```python
from build123d import *

# Parameters (mm, degrees)
SKETCH_1_W           = 206.744673609
SKETCH_1_H           = 106.97480061
EXTRUDE_1_DEPTH      = 3
SKETCH_3_W           = 200.744673609
SKETCH_3_H           = 100.97480061
EXTRUDE_2_DEPTH      = 22.6000508
SKETCH_4_W           = 18
SKETCH_4_H           = 10
CUT_EXTRUDE_1_DEPTH  = 5
SKETCH_6_W           = 16
SKETCH_6_H           = 16
CUT_EXTRUDE_2_DEPTH  = 5
SKETCH_7_W           = 16
SKETCH_7_H           = 16
CUT_EXTRUDE_3_DEPTH  = 5
SKETCH_8_W           = 18
SKETCH_8_H           = 10
CUT_EXTRUDE_4_DEPTH  = 5
SKETCH_9_W           = 35.828584262
SKETCH_9_H           = 13.394073463
CUT_EXTRUDE_5_DEPTH  = 5
SKETCH_10_R          = 3.719289999
CUT_EXTRUDE_6_DEPTH  = 5
SKETCH_11_W          = 9.469470229
SKETCH_11_H          = 12.194282659
CUT_EXTRUDE_7_DEPTH  = 5
SKETCH_12_R          = 3.134321658
CUT_EXTRUDE_8_DEPTH  = 5
SKETCH_13_R          = 1.6
CUT_EXTRUDE_9_DEPTH  = 5
SKETCH_15_W          = 25
SKETCH_15_H          = 20
CUT_EXTRUDE_11_DEPTH = 1.5
SKETCH_16_W          = 20
SKETCH_16_H          = 70
CUT_EXTRUDE_12_DEPTH = 1.5
FILLET_1_R           = 1.5
SKETCH_17_W          = 18.030255685
SKETCH_17_H          = 1.793339536
SKETCH_17_W_2        = 18.10659189
SKETCH_17_W_3        = 18.089855477
SKETCH_17_W_4        = 17.999756417
SKETCH_17_W_5        = 18.030454167
CUT_EXTRUDE_13_DEPTH = 6.89172601
SKETCH_18_W          = 18.338169952
SKETCH_18_H          = 1.939199609
CUT_EXTRUDE_14_DEPTH = 7.158781029
SKETCH_21_W          = 7.461807672
SKETCH_21_H          = 3.5
SKETCH_21_W_2        = 3.5
SKETCH_21_H_2        = 6.158755504
SKETCH_21_H_3        = 6.106655877
SKETCH_21_H_4        = 6.247919092
CUT_EXTRUDE_16_DEPTH = 13


with BuildPart() as part:
    # 草图1 → 凸台-拉伸1 (new body)
    with BuildSketch(Plane(origin=(0, 0, -6), x_dir=(-1, 0, 0), z_dir=(0, 0, -1))):
        with Locations((-142.557122174, -194.856389383)):
            Rectangle(SKETCH_1_W, SKETCH_1_H)
    extrude(amount=EXTRUDE_1_DEPTH)

    # 草图3 → 凸台-拉伸2 (add)
    with BuildSketch(Plane.XY.offset(-6)):
        Polygon((39.18478537, -141.368989078), (245.929458979, -141.368989078), (245.929458979, -248.343789688), (39.18478537, -248.343789688), (39.18478537, -243.18233024), (39.18478537, -146.483402372), align=None)
        with Locations((142.557122174, -194.856389383)):
            Rectangle(SKETCH_3_W, SKETCH_3_H, mode=Mode.SUBTRACT)
    extrude(amount=EXTRUDE_2_DEPTH)

    # 草图4 → 切除-拉伸1 (cut)
    with BuildSketch(Plane.XZ.offset(248.343789688)):
        with Locations((105.2106038, 4.708324791)):
            Rectangle(SKETCH_4_W, SKETCH_4_H)
        with Locations((63.5106038, 4.708324791)):
            Rectangle(SKETCH_4_W, SKETCH_4_H)
        with Locations((147.8106038, 4.708324791)):
            Rectangle(SKETCH_4_W, SKETCH_4_H)
        with Locations((190.5106038, 4.708324791)):
            Rectangle(SKETCH_4_W, SKETCH_4_H)
        with Locations((233.2106038, 4.708324791)):
            Rectangle(SKETCH_4_W, SKETCH_4_H)
    extrude(amount=-CUT_EXTRUDE_1_DEPTH, mode=Mode.SUBTRACT)

    # 草图6 → 切除-拉伸2 (cut)
    with BuildSketch(Plane(origin=(245.929458979, 0, 0), x_dir=(0, 0, -1), z_dir=(1, 0, 0))):
        with Locations((-6.6000508, -220.799301723)):
            Rectangle(SKETCH_6_W, SKETCH_6_H)
        with Locations((-6.6000508, -197.299301723)):
            Rectangle(SKETCH_6_W, SKETCH_6_H)
        with Locations((-6.6000508, -173.799301723)):
            Rectangle(SKETCH_6_W, SKETCH_6_H)
    extrude(amount=-CUT_EXTRUDE_2_DEPTH, mode=Mode.SUBTRACT)

    # 草图7 → 切除-拉伸3 (cut)
    with BuildSketch(Plane(origin=(0, -141.368989078, 0), x_dir=(1, 0, 0), z_dir=(0, 1, 0))):
        with Locations((226.905896319, -6.6000508)):
            Rectangle(SKETCH_7_W, SKETCH_7_H)
    extrude(amount=-CUT_EXTRUDE_3_DEPTH, mode=Mode.SUBTRACT)

    # 草图8 → 切除-拉伸4 (cut)
    with BuildSketch(Plane(origin=(0, -141.368989078, 0), x_dir=(1, 0, 0), z_dir=(0, 1, 0))):
        with Locations((143.087906607, -4.441269771)):
            Rectangle(SKETCH_8_W, SKETCH_8_H)
    extrude(amount=-CUT_EXTRUDE_4_DEPTH, mode=Mode.SUBTRACT)

    # 草图9 → 切除-拉伸5 (cut)
    with BuildSketch(Plane(origin=(0, -141.368989078, 0), x_dir=(1, 0, 0), z_dir=(0, 1, 0))):
        with Locations((193.834394064, -4.192873823)):
            Rectangle(SKETCH_9_W, SKETCH_9_H)
    extrude(amount=-CUT_EXTRUDE_5_DEPTH, mode=Mode.SUBTRACT)

    # 草图10 → 切除-拉伸6 (cut)
    with BuildSketch(Plane(origin=(0, -141.368989078, 0), x_dir=(1, 0, 0), z_dir=(0, 1, 0))):
        with Locations(Location((101.045841124, -4.188653157, 0), (0, 0, 270))):
            Circle(SKETCH_10_R)
    extrude(amount=-CUT_EXTRUDE_6_DEPTH, mode=Mode.SUBTRACT)

    # 草图11 → 切除-拉伸7 (cut)
    with BuildSketch(Plane(origin=(0, -141.368989078, 0), x_dir=(1, 0, 0), z_dir=(0, 1, 0))):
        with Locations((57.128440025, -10.502909471)):
            Rectangle(SKETCH_11_W, SKETCH_11_H)
    extrude(amount=-CUT_EXTRUDE_7_DEPTH, mode=Mode.SUBTRACT)

    # 草图12 → 切除-拉伸8 (cut)
    with BuildSketch(Plane.ZY.offset(-39.18478537)):
        with Locations((4.250612207, -173.693029578)):
            Circle(SKETCH_12_R)
        with Locations((4.250612207, -197.243029578)):
            Circle(SKETCH_12_R)
        with Locations((4.250612207, -220.793029578)):
            Circle(SKETCH_12_R)
    extrude(amount=-CUT_EXTRUDE_8_DEPTH, mode=Mode.SUBTRACT)

    # 草图13 → 切除-拉伸9 (cut)
    with BuildSketch(Plane(origin=(0, 0, -9), x_dir=(-1, 0, 0), z_dir=(0, 0, -1))):
        with Locations((-238.585543847, -149.289415757)):
            Circle(SKETCH_13_R)
        with Locations((-46.99814318, -148.85706783)):
            Circle(SKETCH_13_R)
        with Locations((-46.669564212, -229.041899724)):
            Circle(SKETCH_13_R)
        with Locations((-239.137231318, -229.121228359)):
            Circle(SKETCH_13_R)
    extrude(amount=-CUT_EXTRUDE_9_DEPTH, mode=Mode.SUBTRACT)

    # 草图15 → 切除-拉伸11 (cut)
    with BuildSketch(Plane(origin=(0, -141.368989078, 0), x_dir=(1, 0, 0), z_dir=(0, 1, 0))):
        with Locations((101.081540793, -4.6000508)):
            Rectangle(SKETCH_15_W, SKETCH_15_H)
    extrude(amount=-CUT_EXTRUDE_11_DEPTH, mode=Mode.SUBTRACT)

    # 草图16 → 切除-拉伸12 (cut)
    with BuildSketch(Plane.ZY.offset(-39.18478537)):
        with Locations((4.6000508, -197.704987162)):
            Rectangle(SKETCH_16_W, SKETCH_16_H)
    extrude(amount=-CUT_EXTRUDE_12_DEPTH, mode=Mode.SUBTRACT)

    # 圆角1
    fillet_1_edges = [part.edges().sort_by_distance(p)[0] for p in [
        (245.929458979, -141.368989078, 3.8000254),
        (39.18478537, -141.368989078, 3.8000254),
        (39.18478537, -248.343789688, 3.8000254),
        (245.929458979, -248.343789688, 3.8000254),
    ]]
    fillet(fillet_1_edges, radius=FILLET_1_R)

    # 草图17 → 切除-拉伸13 (cut)
    with BuildSketch(Plane.XY.offset(16.6000508)):
        with Locations((63.500922097, -246.240459456)):
            Rectangle(SKETCH_17_W, SKETCH_17_H)
        with Locations((105.179998956, -246.240459456)):
            Rectangle(SKETCH_17_W_2, SKETCH_17_H)
        with Locations((147.809231135, -246.240459456)):
            Rectangle(SKETCH_17_W_3, SKETCH_17_H)
        with Locations((190.556004567, -246.240459456)):
            Rectangle(SKETCH_17_W_4, SKETCH_17_H)
        with Locations((233.233676321, -246.240459456)):
            Rectangle(SKETCH_17_W_5, SKETCH_17_H)
    extrude(amount=-CUT_EXTRUDE_13_DEPTH, mode=Mode.SUBTRACT)

    # 草图18 → 切除-拉伸14 (cut)
    with BuildSketch(Plane.XY.offset(16.6000508)):
        with Locations((143.227232083, -143.399389273)):
            Rectangle(SKETCH_18_W, SKETCH_18_H)
    extrude(amount=-CUT_EXTRUDE_14_DEPTH, mode=Mode.SUBTRACT)

    # 草图21 → 切除-拉伸16 (cut)
    with BuildSketch(Plane.XY.offset(16.6000508)):
        with Locations((101.01663333, -143.118989078)):
            Rectangle(SKETCH_21_W, SKETCH_21_H)
        with Locations((40.93478537, -173.649755278)):
            Rectangle(SKETCH_21_W_2, SKETCH_21_H_2)
        with Locations((40.93478537, -197.254331907)):
            Rectangle(SKETCH_21_W_2, SKETCH_21_H_3)
        with Locations((40.93478537, -220.776300492)):
            Rectangle(SKETCH_21_W_2, SKETCH_21_H_4)
    extrude(amount=-CUT_EXTRUDE_16_DEPTH, mode=Mode.SUBTRACT)


solid = part.part
```
The model under review builds one solid part; all positions refer to its coordinate system, in mm. A direction names the side the tool comes from. Round coordinates to 2 decimals unless told otherwise and drop trailing zeros. Loops run counter-clockwise (first coordinate to the right, second up) from the corner with the lowest first, then second, coordinate; pieces in that order, holes last. Notation, with made-up numbers: M -36.75,38.25 L 5.25,38.25 A22 ccw 5.25,50.25 Z; hole C 14.5,-27.75 d6. An arc over 180 degrees is marked long. Write item = value, one per line.
Item 1: Take a section at D-D on y = -220. Write out the cut boundary in (x, z).
Return value:
outline = M 39.18,-9 L 245.93,-9 L 245.93,-1.4 L 242.93,-1.4 L 242.93,-6 L 42.18,-6 L 42.18,1.22 L 40.68,1.22 L 40.68,-5.4 L 39.18,-5.4 Z; M 242.93,14.6 L 245.93,14.6 L 245.93,16.6 L 242.93,16.6 Z
Item 2: For line 1 (X direction, y = -243, z = 13.25); line 2 (Y direction, x = 156, z = -3.75); line 3 (Y direction, x = 91.5, z = -2.25), list the stretches that pass through material, from the lowest coordinate up. Write a range as [from, to].
Return value:
line_1 = [39.18, 42.18], [242.93, 245.93]
line_2 = [-248.34, -245.34], [-144.37, -141.37]
line_3 = [-248.34, -245.34], [-144.37, -142.87]
Item 3: Insertion check: P1, Ø0.9, axis at x = 40.5, z = 11.5, coming from the +Y side; P2, Ø5, axis at y = -216, z = 12, coming from the -X side. Each pin has a flat end and moves straight along its axis. Give the tip position at first contact, or say it passes through.
Return value:
P1 = -141.37
P2 = 40.68
Item 4: Take a section at C-C on y = -241.5. Write out the cut boundary in (x, z).
Return value:
outline = M 39.18,-9 L 245.93,-9 L 245.93,16.6 L 242.93,16.6 L 242.93,-6 L 42.18,-6 L 42.18,16.6 L 39.18,16.6 Z
Item 5: The part is to be moulded in two halves that separate along Y. For faces 6 (the flat face through (119, -245.344, 3)), 7 (the flat face through (144, -194, -9)), 8 (the flat face through (144, -248.344, -2)), 9 (the flat face through (118, -141.369, 4)), say which applies: released by +Y, released by -Y, zero draft, split by the parting line, or undercut.
Return value:
face_6 = undercut
face_7 = zero draft
face_8 = released by -Y
face_9 = released by +Y
Item 6: Take a section at A-A on y = -202.5. Write out the cut boundary in (x, z).
Return value:
outline = M 39.18,-9 L 245.93,-9 L 245.93,-1.4 L 242.93,-1.4 L 242.93,-6 L 42.18,-6 L 42.18,16.6 L 39.18,16.6 L 39.18,14.6 L 40.68,14.6 L 40.68,-5.4 L 39.18,-5.4 Z; M 242.93,14.6 L 245.93,14.6 L 245.93,16.6 L 242.93,16.6 Z
Item 7: Take a section at B-B on x = 191.5. Write out the cut boundary in (y, z), then the cut area to 3 significant figures.
Return value:
outline = M -248.34,-9 L -141.37,-9 L -141.37,-2.5 L -144.37,-2.5 L -144.37,-6 L -245.34,-6 L -245.34,-0.29 L -248.34,-0.29 Z; M -248.34,9.71 L -247.14,9.71 L -247.14,16.6 L -248.34,16.6 Z; M -144.37,10.89 L -141.37,10.89 L -141.37,16.6 L -144.37,16.6 Z
area = 374 mm2
Item 8: Machinability: for faces 1 (the flat face through (101, -142.869, 0)), 2 (the flat face through (63, -247.137, 13)), 3 (the flat face through (42, -152, 16.6)), 4 (the cylindrical face through (41.42, -197.11, 1.12)), 5 (the flat face through (40.685, -197, 0)), which of the approach directions +Z, -Z, +X, -X, +Y, -Y give a long, thin tool a straight path to every point of the face, cutting with its end or side? Answer none if there is none.
Return value:
face_1 = +Y
face_2 = +Z
face_3 = +Z, +X, -X, +Y, -Y
face_4 = +X, -X
face_5 = -X
